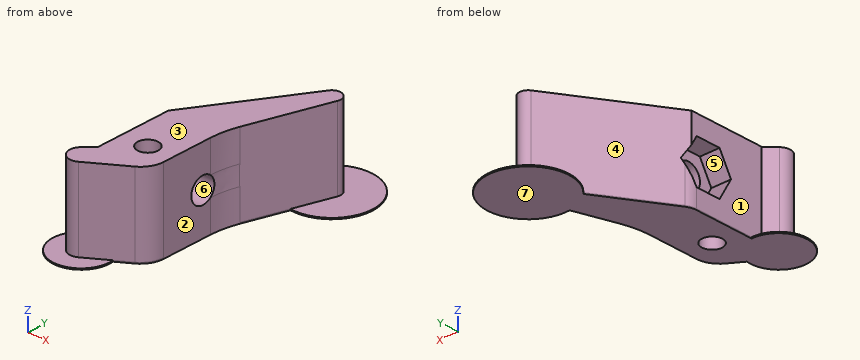
```python
from build123d import *

# Parameters (mm, degrees)
BOSS_EXTRUDE1_DEPTH        = 13.799999061
BOSS_EXTRUDE2_DEPTH        = 0.2
CUT_EXTRUDE1_DEPTH         = 3.400001203
F_4_3_4_3_DIAMETER_HOLE1_D = 4.3
FILLET1_R                  = 3
FILLET2_R                  = 4
FILLET3_R                  = 15
SKETCH8_R                  = 1.75
CUT_EXTRUDE2_DEPTH         = 50.443502835


with BuildPart() as part:
    # Sketch1 → Boss-Extrude1 (new body)
    with BuildSketch(Plane.XY.offset(36.05999958)):
        with BuildLine():
            Line((32.485525439, 18.054212076), (21.200000344, 0.318097361))
            Line((21.200000344, 0.318097361), (21.200000344, -12.753243365))
            Line((21.200000344, -12.753243365), (19.621141825, -14.332101884))
            ThreePointArc((19.621141825, -14.332101884), (19.48110052, -16.933843676), (22.052777974, -17.352349348))
            Line((22.052777974, -17.352349348), (30.004000079, -12.252479732))
            Line((30.004000079, -12.252479732), (30.004000079, 1.043246227))
            Line((30.004000079, 1.043246227), (35.17606489, 16.780626974))
            ThreePointArc((35.17606489, 16.780626974), (34.392817656, 18.604732161), (32.485525439, 18.054212076))
        make_face()
    extrude(amount=-BOSS_EXTRUDE1_DEPTH)

    # Sketch2 → Boss-Extrude2 (add)
    with BuildSketch(Plane(origin=(0, 0, 22.260000519), x_dir=(-1, 0, 0), z_dir=(0, 0, -1))):
        with BuildLine():
            Line((-28.814945272, 12.285604299), (-21.19999872, 0.318097361))
            Line((-21.19999872, 0.318097361), (-21.19999872, -10.863853544))
            ThreePointArc((-21.19999872, -10.863853544), (-17.77320484, -19.33342263), (-25.791833238, -14.954140106))
            Line((-25.791833238, -14.954140106), (-30.004000079, -12.252479732))
            Line((-30.004000079, -12.252479732), (-30.004000079, 1.043246227))
            Line((-30.004000079, 1.043246227), (-33.041298024, 10.285031848))
            ThreePointArc((-33.041298024, 10.285031848), (-36.745962089, 23.575923167), (-28.814945272, 12.285604299))
        make_face()
    extrude(amount=BOSS_EXTRUDE2_DEPTH)

    # Sketch3 → Cut-Extrude1 (cut)
    with BuildSketch(Plane.ZY.offset(-21.200000344)):
        Polygon((29.060742246, -7.024871659), (32.760371092, -4.888032935), (32.759628896, -0.615641007), (29.059257854, 1.519912196), (25.359629008, -0.616926528), (25.360371203, -4.889318456), align=None)
    extrude(amount=-CUT_EXTRUDE1_DEPTH, mode=Mode.SUBTRACT)

    # Ø4.3 (4.3) Diameter Hole1 (through all)
    with Locations(Plane.ZY.offset(-24.600001547)):
        with Locations((29.06000005, -2.752479732)):
            Hole(F_4_3_4_3_DIAMETER_HOLE1_D / 2)

    # Fillet1
    fillet1_edges = [part.edges().sort_by_distance(p)[0] for p in [
        (21.200000344, 0.318097361, 24.619244439),
        (21.19999872, 0.318097361, 22.160000519),
    ]]
    fillet(fillet1_edges, radius=FILLET1_R)

    # Fillet2
    fillet2_edges = [part.edges().sort_by_distance(p)[0] for p in [
        (30.004000079, -12.252479732, 29.06000005),
    ]]
    fillet(fillet2_edges, radius=FILLET2_R)

    # Fillet3
    fillet3_edges = [part.edges().sort_by_distance(p)[0] for p in [
        (30.004000079, 1.043246227, 29.06000005),
    ]]
    fillet(fillet3_edges, radius=FILLET3_R)

    # Sketch8 → Cut-Extrude2 (cut, through all)
    with BuildSketch(Plane.XY.offset(36.05999958)):
        with Locations((25.700000344, -8.352349348)):
            Circle(SKETCH8_R)
    extrude(amount=-CUT_EXTRUDE2_DEPTH, mode=Mode.SUBTRACT)


solid = part.part
```
The model under review builds one solid part; all positions refer to its coordinate system, in mm. Face numbers are marked on the shaded views. A direction names the side the tool comes from. Round coordinates to 2 decimals unless told otherwise and drop trailing zeros. Order: outer loops, then holes, each group sorted by start corner. A loop starts at its lowest first (then second) coordinate and runs counter-clockwise, first axis right, second up. Notation, with made-up numbers: M 82.25,17 L 86.25,17 A14 cw 86.25,22 Z; hole C -34,42 d2. An arc over 180 degrees is marked long. Use a Markdown table: item, result.
1) Consider section B-B (x = 31.25). Write out the cut boundary in (y, z).
Report:
| item | result |
|---|---|
| outline | M 4.83,22.06 L 23.79,22.06 L 23.79,22.26 L 16.11,22.26 L 16.11,36.06 L 4.83,36.06 Z |
2) Tool access review of the marked faces 1, 2 and 3: name each direction out of +Z, -Z, +X, -X, +Y, -Y from which nothing blocks a thin tool from reaching the whole face with its end or side.
Report:
| item | result |
|---|---|
| face 1 | +Z, -X, +Y |
| face 2 | +Z, -Z, +X, -Y |
| face 3 | +Z, +X, -X, +Y, -Y |
3) Insertion check: pin 1 (2.5 mm diameter, centred on y = -4, z = 27.5, fed in from +X); pin 2 (1.5 mm diameter, centred on x = 28, z = 29.5, fed in from +Y); pin 3 (1 mm diameter, centred on x = 29, z = 24, fed in from +Y). Each pin has a flat end and moves straight along its axis. Give the tip position at first contact, or say it passes through.
Report:
| item | result |
|---|---|
| pin 1 | x = 30 |
| pin 2 | y = 12.18 |
| pin 3 | y = 13.36 |
4) Consider section C-C (y = 17.5). Write out the cut boundary in (x, z), then the cut area to 3 significant figures.
Report:
| item | result |
|---|---|
| outline | M 26.76,22.06 L 40.75,22.06 L 40.75,22.26 L 35.23,22.26 L 35.23,36.06 L 32.13,36.06 L 32.13,22.26 L 26.76,22.26 Z |
| area | 45.5 mm^2 |
5) Wall thickness on line 1 along Y through (x, z) = (26.5, 27.5); line 2 along Y through (x, z) = (25.7, 30.5); line 3 along X through (y, z) = (-8.5, 29): over which ranges is each line inside the solid? List them lowest first. Write a range as [from, to].
Report:
| item | result |
|---|---|
| line 1 | [-14.5, -9.91], [-6.8, -4.23], [-1.27, 8.65] |
| line 2 | [-15.01, -10.1], [-6.6, -4.35], [-1.16, 7.39] |
| line 3 | [21.2, 23.96], [27.44, 30] |
6) Draft analysis for pull direction Y (two halves, no side actions). For the marked faces 4, 5, 6 and 7, state which applies: released by +Y, released by -Y, zero draft, split by the parting line, or undercut.
Report:
| item | result |
|---|---|
| face 4 | released by +Y |
| face 5 | undercut |
| face 6 | undercut |
| face 7 | zero draft |
7) Consider section A-A (z = 23.75). Write out the cut boundary in (x, y), then the cut area to 3 significant figures.
Report:
| item | result |
|---|---|
| outline | M 19.62,-14.33 A1.95 ccw 22.05,-17.35 L 28.16,-13.43 A4 ccw 30,-10.07 L 30,-1.36 A15 cw 30.75,3.32 L 35.18,16.78 A1.5 ccw 32.49,18.05 L 21.67,1.06 A3 ccw 21.2,-0.56 L 21.2,-12.75 Z; hole C 25.7,-8.35 d3.5 |
| area | 237 mm^2 |
